```python
from build123d import *

# Parameters (mm, degrees)
SKETCH1_R                  = 2.75
SKETCH1_W                  = 130
SKETCH1_H                  = 38
BOSS_EXTRUDE1_DEPTH        = 10
SKETCH1_2_W                = 130
SKETCH1_2_H                = 38
BOSS_EXTRUDE2_DEPTH        = 10
M3_5_CLEARANCE_HOLE1_D     = 4.8
M3_5_CLEARANCE_HOLE1_DEPTH = 8
M3_5_CLEARANCE_HOLE1_TIP   = 1.442065486
CUT_EXTRUDE1_DEPTH         = 10
M16_CLEARANCE_HOLE1_D      = 19
M16_CLEARANCE_HOLE1_DEPTH  = 6
M8_CLEARANCE_HOLE1_D       = 9


with BuildPart() as part:
    # Sketch1 → Boss-Extrude1 (new body)
    with BuildSketch(Plane(origin=(0, 0, 0), x_dir=(1, 0, 0), z_dir=(0, 1, 0))):
        with BuildLine():
            Line((67, 30), (-67, 30))
            ThreePointArc((-67, 30), (-69.121320344, 29.121320344), (-70, 27))
            Line((-70, 27), (-70, -27))
            ThreePointArc((-70, -27), (-69.121320344, -29.121320344), (-67, -30))
            Line((-67, -30), (67, -30))
            ThreePointArc((67, -30), (69.121320344, -29.121320344), (70, -27))
            Line((70, -27), (70, 27))
            ThreePointArc((70, 27), (69.121320344, 29.121320344), (67, 30))
        make_face()
        with Locations(Location((-60, 24, 0), (0, 0, 270))):
            Circle(SKETCH1_R, mode=Mode.SUBTRACT)
        with Locations(Location((-60, -24, 0), (0, 0, 270))):
            Circle(SKETCH1_R, mode=Mode.SUBTRACT)
        with Locations(Location((60, -24, 0), (0, 0, 270))):
            Circle(SKETCH1_R, mode=Mode.SUBTRACT)
        with Locations(Location((60, 24, 0), (0, 0, 270))):
            Circle(SKETCH1_R, mode=Mode.SUBTRACT)
        Rectangle(SKETCH1_W, SKETCH1_H, mode=Mode.SUBTRACT)
    extrude(amount=BOSS_EXTRUDE1_DEPTH)

    # Sketch1<2> → Boss-Extrude2 (add)
    with BuildSketch(Plane(origin=(0, 0, 0), x_dir=(1, 0, 0), z_dir=(0, 1, 0))):
        Rectangle(SKETCH1_2_W, SKETCH1_2_H)
    extrude(amount=BOSS_EXTRUDE2_DEPTH)

    # M3.5 Clearance Hole1
    with Locations(Plane(origin=(0, 10, 0), x_dir=(1, 0, 0), z_dir=(0, 1, 0))):
        with Locations((0, 0), (-15.181752664, -15.463217926), (15.181752664, 15.463217926), (15.181752664, -15.463217926), (-15.181752664, 15.463217926)):
            Hole(M3_5_CLEARANCE_HOLE1_D / 2, depth=M3_5_CLEARANCE_HOLE1_DEPTH)
            with Locations((0, 0, -(M3_5_CLEARANCE_HOLE1_DEPTH + M3_5_CLEARANCE_HOLE1_TIP / 2))):  # 118° drill point
                Cone(0, M3_5_CLEARANCE_HOLE1_D / 2, M3_5_CLEARANCE_HOLE1_TIP, mode=Mode.SUBTRACT)

    # Sketch6 → Cut-Extrude1 (cut)
    with BuildSketch(Plane(origin=(0, 10, 0), x_dir=(1, 0, 0), z_dir=(0, 1, 0))):
        with BuildLine():
            Line((-30, 10), (30, 10))
            ThreePointArc((30, 10), (40, 0), (30, -10))
            Line((30, -10), (-30, -10))
            ThreePointArc((-30, -10), (-40, 0), (-30, 10))
        make_face()
    extrude(amount=-CUT_EXTRUDE1_DEPTH, mode=Mode.SUBTRACT)

    # M16 Clearance Hole1
    with Locations(Plane(origin=(0, 0, 0), x_dir=(-1, 0, 0), z_dir=(0, -1, 0))):
        with Locations((0, 0), (-45, -15), (45, 15), (45, -15), (-45, 15)):
            Hole(M16_CLEARANCE_HOLE1_D / 2, depth=M16_CLEARANCE_HOLE1_DEPTH)

    # M8 Clearance Hole1 (through all)
    with Locations(Plane(origin=(0, 0, 0), x_dir=(-1, 0, 0), z_dir=(0, -1, 0))):
        with Locations((45, -15), (45, 15), (-45, 15), (-45, -15)):
            Hole(M8_CLEARANCE_HOLE1_D / 2)


solid = part.part
```
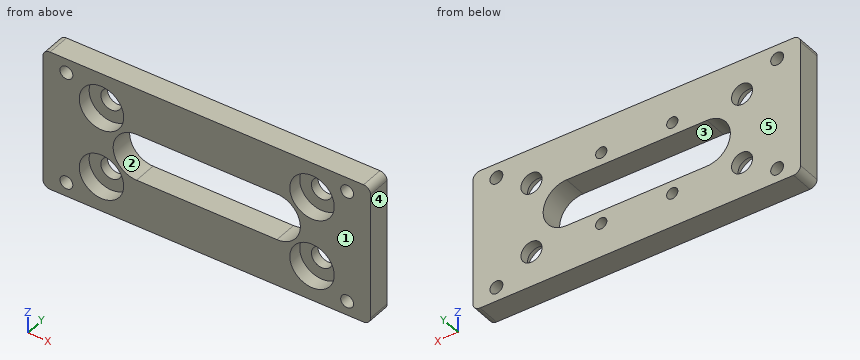
Design review of the part built by this model. Coordinates are the model's own, in mm. Face numbers are marked on the shaded views. A direction names the side the tool comes from. Coordinates: 2 decimals unless noted, no trailing zeros. Order: outer loops, then holes, each group sorted by start corner. A loop starts at its lowest first (then second) coordinate and runs counter-clockwise, first axis right, second up. Notation, with made-up numbers: (-22, 13.5) - (18, 13.5) arc R22 ccw to (18, 32.5) - close; hole circle Ø5 at (79.25, 19.25). An arc over 180 degrees is marked (long way). One line per question, with ' | ' between items.
Q1. Consider section A-A, the plane x = -25. Give the boundary of the cut face in (y, z), then the cut area to 3 significant figures.
Answer key:
outline: (0, -30) - (10, -30) - (10, -10) - (0, -10) - close; (0, 10) - (10, 10) - (10, 30) - (0, 30) - close | area: 400 mm2
Q2. Consider section B-B, the plane z = -2.5. Give the boundary of the cut face in (x, y).
Answer key:
outline: (-70, 0) - (-39.68, 0) - (-39.68, 10) - (-70, 10) - close; (39.68, 0) - (70, 0) - (70, 10) - (39.68, 10) - close
Q3. To check wall thickness, follow line 1 along X through (y, z) = (7.5, -24); line 2 along Z through (x, y) = (45, 9.1); line 3 along X through (y, z) = (5.5, 9). State the ranges of each line that lie inside material, in increasing order.
Answer key:
line 1: x = -70 to -62.75, -57.25 to 57.25, 62.75 to 70 | line 2: z = -30 to -19.5, -10.5 to 10.5, 19.5 to 30 | line 3: x = -70 to -52.37, -37.63 to -34.36, 34.36 to 37.63, 52.37 to 70
Q4. Consider section C-C, the plane x = 45. Give the boundary of the cut face in (y, z).
Answer key:
outline: (0, -30) - (10, -30) - (10, -19.5) - (6, -19.5) - (6, -24.5) - (0, -24.5) - close; (0, -5.5) - (6, -5.5) - (6, -10.5) - (10, -10.5) - (10, 10.5) - (6, 10.5) - (6, 5.5) - (0, 5.5) - close; (0, 24.5) - (6, 24.5) - (6, 19.5) - (10, 19.5) - (10, 30) - (0, 30) - close
Q5. The part is to be moulded in two halves that separate along X. For the marked faces 3, 4 and 5, say which applies: +X half, -X half, draft (parallel to the pull), parting line (faces both ways), or undercut.
Answer key:
face 3: undercut | face 4: +X half | face 5: draft
Q6. For the marked faces 1 and 2, list the 3-axis set-ups (+Z, -Z, +X, -X, +Y, -Y) from which the entire face can be reached by the end or side of a thin tool; tool diameter is ignored.
Answer key:
face 1: +Z, -Z, +X, -X, -Y | face 2: +Y, -Y
Q7. Consider section D-D, the plane y = 8.5. Give the number of separate pieces and of enclosed holes in the cut face, then the cut area to 3 significant figures.
Answer key:
separate pieces: 1 | enclosed holes: 13 | area: 6,460 mm2
Q8. Clearance check with flat-ended pins moving along their axes: pin 1 Ø3 at (x, z) = (-31.5, 9) entering from +Y; pin 2 Ø5.5 at (x, z) = (-48, 14) entering from -Y; pin 3 Ø4 at (x, z) = (15.18, 15.46) entering from +Y. State where each tip first meets the part, or that it passes through.
Answer key:
pin 1: stops at y = 10 | pin 2: stops at y = 6 | pin 3: stops at y = 1.76
